CAD build for the part. Positions are in the model's coordinates, mm. A direction names the side the tool comes from. Coordinates: 2 decimals unless noted, no trailing zeros. Write each loop counter-clockwise with the first axis right and the second up, starting at its lowest first coordinate (ties: lowest second). Pieces come first, ordered by that corner, then holes. Notation, with made-up numbers: (-24.75, 5) -> (24.25, 5) arc R15 ccw to (24.25, 13) -> close; hole circle Ø5 at (-37.5, 8). An arc over 180 degrees is marked (long way). Answer as CSV lines item,"result".
```python
from build123d import *

# Parameters (mm, degrees)
BOSS_EXTRUDE1_DEPTH = 4.826
FILLET1_R           = 1.27
FILLET2_R           = 2.54


with BuildPart() as part:
    # Sketch1 → Boss-Extrude1 (new body)
    with BuildSketch(Plane(origin=(0, 0, 0), x_dir=(1, 0, 0), z_dir=(0, 1, 0))):
        Polygon((-80.01, 25.4), (-55.000893554, 25.4), (-59.944, 15.69860736), (-56.7755808, 14.084217143), (-51.009901453, 25.4), (-12.7, 25.4), (-12.7, 34.036), (12.7, 34.036), (12.7, 25.4), (51.009901453, 25.4), (56.7755808, 14.084217143), (59.944, 15.69860736), (55.000893554, 25.4), (80.01, 25.4), (80.01, 12.7), (72.644, 12.7), (72.644, -12.7), (80.01, -12.7), (80.01, -25.4), (44.45, -25.4), (44.45, -34.036), (23.876, -34.036), (23.876, -25.4), (-23.876, -25.4), (-23.876, -28.575), (-44.45, -28.575), (-44.45, -25.4), (-80.01, -25.4), (-80.01, -12.7), (-72.644, -12.7), (-72.644, 12.7), (-80.01, 12.7), align=None)
    extrude(amount=BOSS_EXTRUDE1_DEPTH)

    # Fillet1
    fillet1_edges = [part.edges().sort_by_distance(p)[0] for p in [
        (-59.944, 2.413, -15.69860736),
        (-56.7755808, 2.413, -14.084217143),
        (56.7755808, 2.413, -14.084217143),
        (59.944, 2.413, -15.69860736),
    ]]
    fillet(fillet1_edges, radius=FILLET1_R)

    # Fillet2
    fillet2_edges = [part.edges().sort_by_distance(p)[0] for p in [
        (-55.000893554, 2.413, -25.4),
        (-51.009901453, 2.413, -25.4),
        (51.009901453, 2.413, -25.4),
        (55.000893554, 2.413, -25.4),
    ]]
    fillet(fillet2_edges, radius=FILLET2_R)


solid = part.part
```
Item 1: Wall check: line 1 (X direction, y = 1.55, z = -17.5); line 2 (X direction, y = 0.9, z = -20.5); line 3 (X direction, y = 3.3, z = -8). Give the ranges that are in metal, low to high. Write a range as from..to.
Answer below:
line 1,"x = -80.01..-59.03, -55.04..55.04, 59.03..80.01"
line 2,"x = -80.01..-57.5, -53.51..53.51, 57.5..80.01"
line 3,"x = -72.64..72.64"
Item 2: Saw through at C-C on z = 6. Give the cut face in (x, y), and give its area (3 significant figures).
Answer below:
outline,"(-72.64, 0) -> (72.64, 0) -> (72.64, 4.83) -> (-72.64, 4.83) -> close"
area,"701 mm2"
Item 3: Saw through at B-B on x = -16.5. Give the cut face in (y, z), and give its area (3 significant figures).
Answer below:
outline,"(0, -25.4) -> (4.83, -25.4) -> (4.83, 25.4) -> (0, 25.4) -> close"
area,"245 mm2"
Item 4: Saw through at A-A on z = -19. Give the cut face in (x, y).
Answer below:
outline,"(-80.01, 0) -> (-58.26, 0) -> (-58.26, 4.83) -> (-80.01, 4.83) -> close; (-54.27, 0) -> (54.27, 0) -> (54.27, 4.83) -> (-54.27, 4.83) -> close; (58.26, 0) -> (80.01, 0) -> (80.01, 4.83) -> (58.26, 4.83) -> close"
Item 5: Flat gauge pins, fed straight in: pin 1 (1.4 mm diameter, centred on y = 2, z = 2.5, fed in from -X); pin 2 (1.4 mm diameter, centred on x = -54, y = 2.5, fed in from +Z); pin 3 (2.5 mm diameter, centred on x = -26, y = 2, fed in from -Z). Where does each tip first touch, or does it go through?
Answer below:
pin 1,"stops at x = -72.64"
pin 2,"stops at z = 25.4"
pin 3,"stops at z = -25.4"
Item 6: 3-axis set-ups, long thin cutter, end or side, ignore diameter. For faces 1 (the flat face through (-23.876, 2, 27)), 2 (the flat face through (-31, 2, -25.4)), 3 (the flat face through (-62, 2, 25.4)): which of +Z, -Z, +X, -X, +Y, -Y reach the whole face in a straight line?
Answer below:
face 1,"+Z, +Y, -Y"
face 2,"-Z, -X, +Y, -Y"
face 3,"+Z, -X, +Y, -Y"
Item 7: Two-plate mould, pull along X, no slides. Class faces 4 (the flat face through (-53.99, 2.38, -19.55)), 5 (the flat face through (-72.644, 2, 0)), 6 (the flat face through (76, 2, 12.7)): pulls with the +X half, pulls with the -X half, needs draft (parallel to the pull), parting line crosses it, or undercut.
Answer below:
face 4,"undercut"
face 5,"pulls with the -X half"
face 6,"needs draft"
